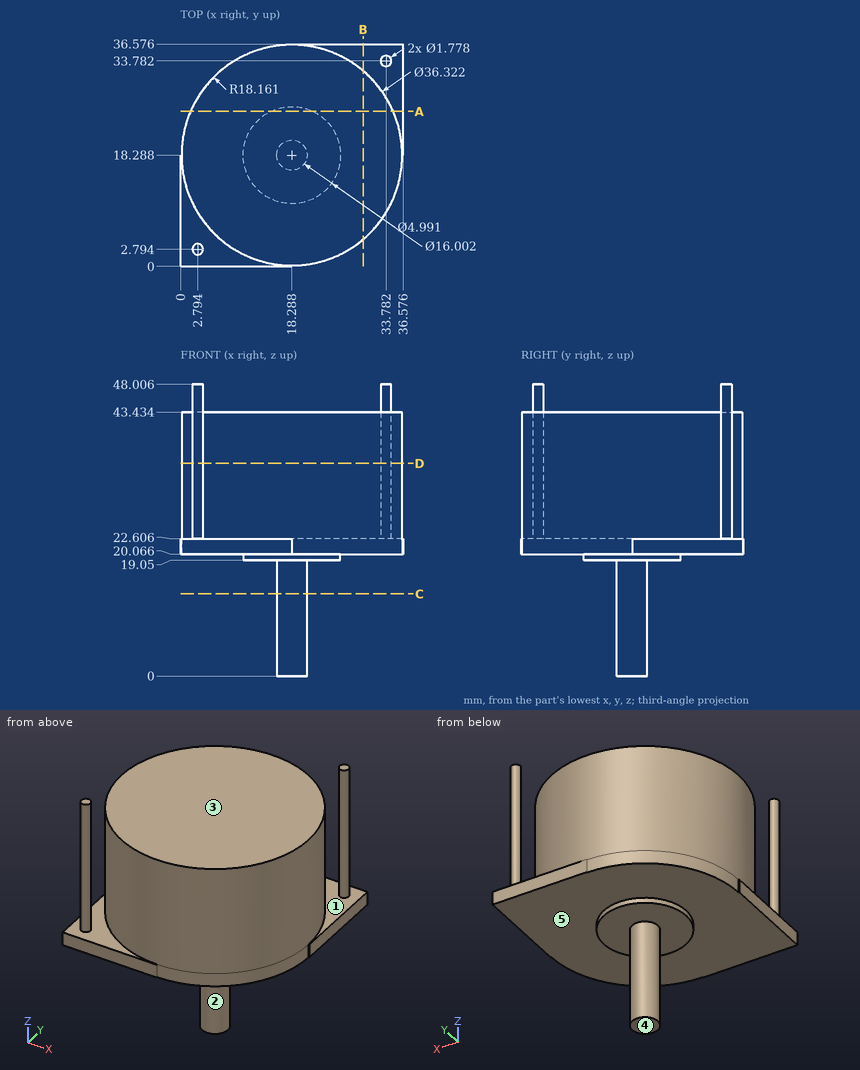
Job drawing, mm, ordinate dimensions from the low corner. One solid piece. A direction names the side the tool comes from. Round coordinates to 2 decimals unless told otherwise and drop trailing zeros. Write each loop counter-clockwise with the first axis right and the second up, starting at its lowest first coordinate (ties: lowest second). Pieces come first, ordered by that corner, then holes.
1) Mould opens along X. For the marked faces 1, 2 and 3 say: +X half, -X half, draft (parallel to the pull), parting line (faces both ways), or undercut.
2) Band-saw the part on D-D, the plane z = 35. List the corners of the cut face in (x, y).
3) Band-saw the part on C-C, the plane z = 13.5. List the corners of the cut face in (x, y).
4) Band-saw the part on B-B, the plane x = 30. List the corners of the cut face in (y, z).
5) Drill centre lines: probe 1 along Z at (x, y) = (18.5, 23); probe 2 along Z at (x, y) = (28.5, 19); probe 3 along Y at (x, z) = (18, 23). Where is each one in solid material? Low to high.
6) Band-saw the part on A-A, the plane y = 25.5. List the corners of the cut face in (x, z).
7) 3-axis set-ups, long thin cutter, end or side, ignore diameter. For the marked faces 4 and 5: which of +Z, -Z, +X, -X, +Y, -Y reach the whole face in a straight line?
8) Pin check, flat tips, straight feed: pin 1 (5 mm diameter, centred on y = 14, z = 10.5, fed in from -X); pin 2 (5 mm diameter, centred on x = 14.5, z = 5, fed in from -Y); pin 3 (17.5 mm diameter, centred on x = 15, y = 18, fed in from -Z); pin 4 (10 mm diameter, centred on y = 19.5, z = 6, fed in from -X). Stop position of each tip, or through.
Ans:
1. face 1: undercut
1. face 2: parting line
1. face 3: draft
2. outline: circle Ø36.32 at (18.29, 18.29); circle Ø1.78 at (2.79, 2.79); circle Ø1.78 at (33.78, 33.78)
3. outline: circle Ø4.99 at (18.29, 18.29)
4. outline: (4.41, 20.07) - (36.58, 20.07) - (36.58, 22.61) - (32.17, 22.61) - (32.17, 43.43) - (4.41, 43.43) - close
5. probe 1: z = 19.05 to 43.43
5. probe 2: z = 20.07 to 43.43
5. probe 3: y = 0.13 to 36.45
6. outline: (1.62, 20.07) - (14.82, 20.07) - (14.82, 19.05) - (21.75, 19.05) - (21.75, 20.07) - (36.58, 20.07) - (36.58, 22.61) - (34.96, 22.61) - (34.96, 43.43) - (1.62, 43.43) - close
7. face 4: -Z, +X, -X, +Y, -Y
7. face 5: -Z
8. pin 1: stops at x = 16.55
8. pin 2: stops at y = 16.15
8. pin 3: stops at z = 0
8. pin 4: stops at x = 15.79
